Geometry: final body of the model. Coordinates: model frame, mm. A direction names the side the tool comes from. Coordinates: 2 decimals unless noted, no trailing zeros. Write each loop counter-clockwise with the first axis right and the second up, starting at its lowest first coordinate (ties: lowest second). Pieces come first, ordered by that corner, then holes. Notation, with made-up numbers: (81.5, 19.5) - (131.5, 19.5) arc R20 ccw to (131.5, 34.5) - close; hole circle Ø7 at (24, -16). An arc over 180 degrees is marked (long way). Put each result on its own line as item: value.
```python
from build123d import *

# Parameters (mm, degrees)
BOSS_EXTRUDE1_DEPTH = 300
SKETCH2_R           = 112.5
SKETCH2_R_2         = 87.5
BOSS_EXTRUDE2_DEPTH = 170
SKETCH3_R           = 37.5
CUT_EXTRUDE3_DEPTH  = 239
CUT_EXTRUDE4_START  = 208
SKETCH5_R           = 25
CUT_EXTRUDE4_DEPTH  = 31


with BuildPart() as part:
    # Sketch1 → Boss-Extrude1 (new body)
    with BuildSketch(Plane.XY):
        with BuildLine():
            Line((-167.5, 0), (167.5, 0))
            ThreePointArc((167.5, 0), (202.855339059, 14.644660941), (217.5, 50))
            Line((217.5, 50), (217.5, 188))
            ThreePointArc((217.5, 188), (223.357864376, 202.142135624), (237.5, 208))
            Line((237.5, 208), (475, 208))
            Line((475, 208), (475, 238))
            Line((475, 238), (237.5, 238))
            ThreePointArc((237.5, 238), (202.144660941, 223.355339059), (187.5, 188))
            Line((187.5, 188), (187.5, 50))
            ThreePointArc((187.5, 50), (181.642135624, 35.857864376), (167.5, 30))
            Line((167.5, 30), (-167.5, 30))
            ThreePointArc((-167.5, 30), (-181.642135624, 35.857864376), (-187.5, 50))
            Line((-187.5, 50), (-187.5, 188))
            ThreePointArc((-187.5, 188), (-202.144660941, 223.355339059), (-237.5, 238))
            Line((-237.5, 238), (-475, 238))
            Line((-475, 238), (-475, 208))
            Line((-475, 208), (-237.5, 208))
            ThreePointArc((-237.5, 208), (-223.357864376, 202.142135624), (-217.5, 188))
            Line((-217.5, 188), (-217.5, 50))
            ThreePointArc((-217.5, 50), (-202.855339059, 14.644660941), (-167.5, 0))
        make_face()
    extrude(amount=BOSS_EXTRUDE1_DEPTH)

    # Sketch2 → Boss-Extrude2 (add)
    with BuildSketch(Plane(origin=(0, 0, 0), x_dir=(1, 0, 0), z_dir=(0, 1, 0))):
        with Locations((0, -150)):
            Circle(SKETCH2_R)
        with Locations((0, -150)):
            Circle(SKETCH2_R_2, mode=Mode.SUBTRACT)
    extrude(amount=BOSS_EXTRUDE2_DEPTH)

    # Sketch3 → Cut-Extrude3 (cut, through all)
    with BuildSketch(Plane(origin=(0, 0, 0), x_dir=(1, 0, 0), z_dir=(0, 1, 0))):
        with Locations((0, -150)):
            Circle(SKETCH3_R)
    extrude(amount=CUT_EXTRUDE3_DEPTH, mode=Mode.SUBTRACT)

    # Sketch5 → Cut-Extrude4 (cut, through all)
    with BuildSketch(Plane(origin=(0, 0, 0), x_dir=(1, 0, 0), z_dir=(0, 1, 0)).offset(CUT_EXTRUDE4_START)):
        with Locations((-355, -150)):
            Circle(SKETCH5_R)
        with Locations((355, -150)):
            Circle(SKETCH5_R)
    extrude(amount=CUT_EXTRUDE4_DEPTH, mode=Mode.SUBTRACT)


solid = part.part
```
1. Section query C-C (z = 150). Count the separate pieces of the cut face and the enclosed holes in it, then the cut area to 3 significant figures.
Answer below:
separate pieces: 4
enclosed holes: 0
area: 40,900 mm²
2. Set-up query: faces 4 (the cylindrical face through (202.536, 223.742, 147.9)), 5 (the flat face through (217.5, 118, 148)), 6 (the flat face through (-38, 30, 149)), 7 (the flat face through (-217.5, 120, 148)). Return all of +Z, -Z, +X, -X, +Y, -Y with unobstructed straight access to the full face (end or side cutting, diameter ignored); none if empty.
Answer below:
face 4: +Z, -Z, +Y
face 5: +Z, -Z, +X, -Y
face 6: +Y
face 7: +Z, -Z, -X, -Y
3. Mould query, pull axis X, two halves, no side actions, for faces 1 (the cylindrical face through (-223.514, 202.297, 147.9)), 2 (the flat face through (187.5, 120, 148)), 3 (the flat face through (-384, 208, 148)). Classes: +X half, -X half, draft (parallel to the pull), parting line (faces both ways), or undercut.
Answer below:
face 1: -X half
face 2: undercut
face 3: draft
4. Section query A-A (y = 155.5). Return loops of the section in (x, z).
Answer below:
outline: (-217.5, 0) - (-187.5, 0) - (-187.5, 300) - (-217.5, 300) - close; circle Ø225 at (0, 150); (187.5, 0) - (217.5, 0) - (217.5, 300) - (187.5, 300) - close; hole circle Ø175 at (0, 150)
5. Section query B-B (x = 355). Return loops of the section in (y, z), then the cut area to 3 significant figures.
Answer below:
outline: (208, 0) - (238, 0) - (238, 125) - (208, 125) - close; (208, 175) - (238, 175) - (238, 300) - (208, 300) - close
area: 7,500 mm²
6. Section query D-D (x = 0). Return loops of the section in (y, z).
Answer below:
outline: (0, 0) - (30, 0) - (30, 37.5) - (170, 37.5) - (170, 62.5) - (30, 62.5) - (30, 112.5) - (0, 112.5) - close; (0, 187.5) - (30, 187.5) - (30, 237.5) - (170, 237.5) - (170, 262.5) - (30, 262.5) - (30, 300) - (0, 300) - close
7. Ray query, probe 1 along X at (y, z) = (131, 150); probe 2 along X at (y, z) = (86.5, 48.5); probe 3 along X at (y, z) = (225, 150). Return the intervals inside material, ascending. Write a range as from..to.
Answer below:
probe 1: x = -217.5..-187.5, -112.5..-87.5, 87.5..112.5, 187.5..217.5
probe 2: x = -217.5..-187.5, -48.52..48.52, 187.5..217.5
probe 3: x = -475..-380, -330..-203.87, 203.87..330, 380..475
8. Pin query (flat end, axial travel): pin 1 Ø12 at (y, z) = (156.5, 264) entering from +X; pin 2 Ø10 at (y, z) = (40.5, 110) entering from +X; pin 3 Ø1.5 at (x, z) = (-313, 187.5) entering from -Y. Return the tip coordinate at first contact, or that it passes through.
Answer below:
pin 1: stops at x = 217.5
pin 2: stops at x = 217.3
pin 3: stops at y = 208
